```python
from build123d import *

# Parameters (mm, degrees)
SKETCH2_R           = 19.05
BOSS_EXTRUDE1_DEPTH = 25.4
CUT_EXTRUDE1_DEPTH  = 38.026544532


with BuildPart() as part:
    # Sketch2 → Boss-Extrude1 (new body)
    with BuildSketch(Plane(origin=(0, 0, 0), x_dir=(1, 0, 0), z_dir=(0, 1, 0))):
        with Locations(Location((0, 0, 0), (0, 0, 270))):
            Circle(SKETCH2_R)
    extrude(amount=BOSS_EXTRUDE1_DEPTH)

    # Sketch4 → Cut-Revolve2 (revolve, cut)
    with BuildSketch(Plane.XY, mode=Mode.PRIVATE) as cut_revolve2_sk:
        with BuildLine():
            Line((-16.51, 15.24), (-19.05, 15.24))
            Line((-19.05, 15.24), (-19.05, 10.16))
            Line((-19.05, 10.16), (-16.51, 10.16))
            ThreePointArc((-16.51, 10.16), (-13.97, 12.7), (-16.51, 15.24))
        make_face()
    revolve(cut_revolve2_sk.sketch.rotate(Axis((0, 0, 0), (0, 1, 0)), 180), axis=Axis((0, 0, 0), (0, 1, 0)), mode=Mode.SUBTRACT)

    # Sketch7 → Cut-Extrude1 (cut, through all)
    with BuildSketch(Plane(origin=(0, 25.4, 0), x_dir=(1, 0, 0), z_dir=(0, 1, 0))):
        Polygon((8.065583261, 0), (4.03279163, 6.985), (-4.03279163, 6.985), (-8.065583261, 0), (-4.03279163, -6.985), (4.03279163, -6.985), align=None)
    extrude(amount=-CUT_EXTRUDE1_DEPTH, mode=Mode.SUBTRACT)


solid = part.part
```
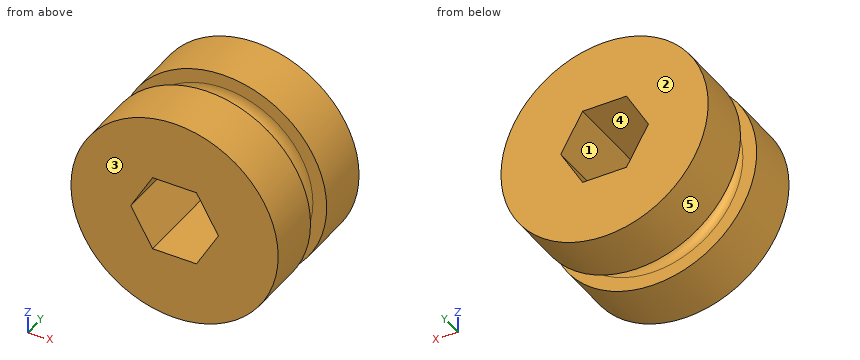
Input: part model. Units: mm. Frame: model coordinates. Face numbers are marked on the shaded views. A direction names the side the tool comes from. Coordinates: 2 decimals unless noted, no trailing zeros. Write each loop counter-clockwise with the first axis right and the second up, starting at its lowest first coordinate (ties: lowest second). Pieces come first, ordered by that corner, then holes. Notation, with made-up numbers: (5.25, -30.75) -> (28.25, -30.75) arc R30 ccw to (28.25, 4.25) -> close; hole circle Ø2 at (-16.5, 26). An arc over 180 degrees is marked (long way). Answer as a JSON object with one key per item and string values.
1. Mould query, pull axis Z, two halves, no side actions, for the marked faces 3, 4 and 5. Classes: released by +Z, released by -Z, zero draft, split by the parting line, or undercut.
Result set:
{"face 3": "zero draft", "face 4": "undercut", "face 5": "split by the parting line"}
2. Section A-A on y = 6.25. Return the cut outline in (x, z) (3 decimals).
Result set:
{"outline": "circle Ø38.1 at (0, 0); hole (-8.066, 0) -> (-4.033, -6.985) -> (4.033, -6.985) -> (8.066, 0) -> (4.033, 6.985) -> (-4.033, 6.985) -> close"}
3. Material intervals for line 1 (Y direction, x = 17.5, z = 3); line 2 (Z direction, x = 0.5, y = 24.5) (3 decimals); line 3 (X direction, y = 16, z = -4.5), sorted ascending. Write a range as from..to.
Result set:
{"line 1": "y = 0..10.16, 15.24..25.4", "line 2": "z = -19.043..-6.985, 6.985..19.043", "line 3": "x = -18.51..-5.47, 5.47..18.51"}
4. Access query for the marked faces 1 and 2. Directions: +Z, -Z, +X, -X, +Y, -Y. A direction counts if a zero-diameter tool reaches every point of the face in a straight line with its end or side. Return the directions, or none.
Result set:
{"face 1": "+Y, -Y", "face 2": "+Z, -Z, +X, -X, +Y"}
5. Section B-B on x = 0. Return the cut outline in (y, z) (3 decimals).
Result set:
{"outline": "(0, -19.05) -> (10.16, -19.05) -> (10.16, -16.51) arc R2.54 cw to (15.24, -16.51) -> (15.24, -19.05) -> (25.4, -19.05) -> (25.4, -6.985) -> (0, -6.985) -> close; (0, 6.985) -> (25.4, 6.985) -> (25.4, 19.05) -> (15.24, 19.05) -> (15.24, 16.51) arc R2.54 cw to (10.16, 16.51) -> (10.16, 19.05) -> (0, 19.05) -> close"}
6. First-contact query: P1, Ø4, axis at y = 19.5, z = 9, coming from the +X side; P2, Ø4, axis at x = -13.5, y = 19, coming from the -Z side; P3, Ø3, axis at y = 9, z = 6, coming from the -X side. Flat tips, straight axial feed; report the tip coordinate or a pass-through.
Result set:
{"P1": "stops at x = 17.72", "P2": "stops at z = -15.19", "P3": "stops at x = -18.51"}
